Input: part model. Units: mm. Frame: model coordinates. A direction names the side the tool comes from. Coordinates: 2 decimals unless noted, no trailing zeros. Write each loop counter-clockwise with the first axis right and the second up, starting at its lowest first coordinate (ties: lowest second). Pieces come first, ordered by that corner, then holes. Notation, with made-up numbers: (42, 53) - (100, 53) arc R19 ccw to (100, 60) - close; hole circle Ø1 at (0, 79). An arc over 180 degrees is marked (long way). Put each result on its own line as item: value. Start each with the question number.
1. Pull-direction query (Z, two-part tool) for faces 1 (the cylindrical face through (-1.25, 0.05, 29.72)), 2 (the flat face through (13, 3, 48)), 3 (the flat face through (14, 0, 50)); classes: released by +Z, released by -Z, zero draft, split by the parting line, or undercut.
2. Line query: line 1 (Z direction, x = -3.5, y = -4.5); line 2 (Y direction, x = 0.5, z = 46); line 3 (X direction, y = -2.75, z = 47.5). Output: solid intervals per line, ascending.
3. Cut plane C-C, the plane z = 9. Return loops of the section in (x, y), and give its area (3 significant figures).
4. Cut plane D-D, the plane x = 18. Return loops of the section in (y, z), and give its area (3 significant figures).
5. Cut plane A-A, the plane y = -2. Return loops of the section in (x, z), and give its area (3 significant figures).
6. Cut plane B-B, the plane x = 3.5. Return loops of the section in (y, z).
7. Access query for faces 4 (the flat face through (13, -3, 48)), 5 (the cylindrical face through (-0.88, -1.72, 47.54)), 6 (the cylindrical face through (27.927, 0.055, 47.535)), 7 (the cylindrical face through (-0.897, 1.677, 47.535)). Directions: +Z, -Z, +X, -X, +Y, -Y. A direction counts if a zero-diameter tool reaches every point of the face in a straight line with its end or side. Return the directions, or none.
8. Pin query (flat end, axial travel): pin 1 (5 mm diameter, centred on y = -3, z = 10.5, fed in from -X); pin 2 (5.5 mm diameter, centred on x = 19, z = 46.5, fed in from -Y); pin 3 (1.5 mm diameter, centred on x = 18.5, z = 46.5, fed in from +Y); pin 4 (8 mm diameter, centred on x = 5.5, z = 40.5, fed in from +Y). Return the tip coordinate at first contact, or that it passes through.
from build123d import *

# Parameters (mm, degrees)
SKETCH_1_R      = 10
EXTRUDE_1_DEPTH = 10
SKETCH_2_R      = 1.25
EXTRUDE_2_DEPTH = 40
EXTRUDE_3_DEPTH = 5


with BuildPart() as part:
    # Эскиз1 → Бобышка-Вытянуть1 (new body)
    with BuildSketch(Plane.XY):
        Circle(SKETCH_1_R)
    extrude(amount=EXTRUDE_1_DEPTH)

    # Эскиз2 → Бобышка-Вытянуть2 (add)
    with BuildSketch(Plane.XY.offset(10)):
        Circle(SKETCH_2_R)
    extrude(amount=EXTRUDE_2_DEPTH)

    # Эскиз3 → Бобышка-Вытянуть3 (add)
    with BuildSketch(Plane.XY.offset(50)):
        with BuildLine():
            Line((0, 3), (25.827062473, 3))
            ThreePointArc((25.827062473, 3), (27.92788481, 0), (25.827062473, -3))
            Line((25.827062473, -3), (0, -3))
            ThreePointArc((0, -3), (-1.242640687, 0), (0, 3))
        make_face()
    extrude(amount=-EXTRUDE_3_DEPTH)


solid = part.part
Report:
1. face 1: undercut
1. face 2: zero draft
1. face 3: released by +Z
2. line 1: z = 0 to 10
2. line 2: y = -3 to 3
2. line 3: x = -0.23 to 26.36
3. outline: circle Ø20 at (0, 0)
3. area: 314 mm^2
4. outline: (-3, 45) - (3, 45) - (3, 50) - (-3, 50) - close
4. area: 30.0 mm^2
5. outline: (-9.8, 0) - (9.8, 0) - (9.8, 10) - (-9.8, 10) - close; (-0.74, 45) - (27.22, 45) - (27.22, 50) - (-0.74, 50) - close
5. area: 336 mm^2
6. outline: (-9.37, 0) - (9.37, 0) - (9.37, 10) - (-9.37, 10) - close; (-3, 45) - (3, 45) - (3, 50) - (-3, 50) - close
7. face 4: +Z, +X, -X, -Y
7. face 5: +Z, -X, -Y
7. face 6: +Z, -Z, +X
7. face 7: +Z, -X, +Y
8. pin 1: stops at x = -9.98
8. pin 2: stops at y = -3
8. pin 3: stops at y = 3
8. pin 4: passes through
